Source: CAD feature listing. Evaluate the final solid. Frame: model axes, mm. A direction names the side the tool comes from. Give positions to 0.01 mm unless a question says otherwise; leave off trailing zeros. Order: outer loops, then holes, each group sorted by start corner. A loop starts at its lowest first (then second) coordinate and runs counter-clockwise, first axis right, second up.
```python
from build123d import *

# Parameters (mm, degrees)
BOSS_EXTRUDE1_DEPTH = 9.75
BOSS_EXTRUDE2_START = -1
BOSS_EXTRUDE2_DEPTH = 5
BOSS_EXTRUDE3_START = 1
SKETCH3_R           = 1.6
BOSS_EXTRUDE3_DEPTH = 1
BOSS_EXTRUDE4_DEPTH = 0.5


with BuildPart() as part:
    # Sketch1 → Boss-Extrude1 (new body)
    with BuildSketch(Plane(origin=(0, 0, 0), x_dir=(0, 0, -1), z_dir=(1, 0, 0))):
        Polygon((-4.875, -6.875), (-4.875, 5.125), (4.875, 5.125), (4.875, -6.875), (6.625, -6.875), (6.625, 6.875), (-6.625, 6.875), (-6.625, -6.875), align=None)
    extrude(amount=BOSS_EXTRUDE1_DEPTH)

    # Sketch2 → Boss-Extrude2 (add)
    with BuildSketch(Plane.XZ.offset(6.875).offset(BOSS_EXTRUDE2_START)):
        with BuildLine():
            Line((0, 9.925), (0, 4.875))
            Line((0, 4.875), (7.75, 4.875))
            Line((7.75, 4.875), (7.75, 9.925))
            ThreePointArc((7.75, 9.925), (3.875, 13.8), (0, 9.925))
        make_face()
        Polygon((0.584103466, 9.925), (2.229551733, 12.775), (5.520448267, 12.775), (7.165896534, 9.925), (5.520448267, 7.075), (2.229551733, 7.075), align=None, mode=Mode.SUBTRACT)
    boss_extrude2 = extrude(amount=-BOSS_EXTRUDE2_DEPTH)

    # Sketch3 → Boss-Extrude3 (add)
    with BuildSketch(Plane.XZ.offset(5.875).offset(BOSS_EXTRUDE3_START)):
        with BuildLine():
            Line((7.75, 6.625), (7.75, 9.925))
            ThreePointArc((7.75, 9.925), (3.875, 13.8), (0, 9.925))
            Line((0, 9.925), (0, 6.625))
            Line((0, 6.625), (7.75, 6.625))
        make_face()
        with Locations(Location((3.875, 9.925, 0), (0, 0, 90))):
            Circle(SKETCH3_R, mode=Mode.SUBTRACT)
    boss_extrude3 = extrude(amount=-BOSS_EXTRUDE3_DEPTH)

    # Mirror1: Boss-Extrude2, Boss-Extrude3 across plane
    add(boss_extrude2.mirror(Plane.XY))
    add(boss_extrude3.mirror(Plane.XY))

    # Sketch4 → Boss-Extrude4 (add)
    with BuildSketch(Plane.ZY):
        Polygon((-6.625, 6.875), (-6.625, -6.875), (-4.375, -6.875), (-4.375, 4.625), (4.375, 4.625), (4.375, -6.875), (6.625, -6.875), (6.625, 6.875), align=None)
    extrude(amount=-BOSS_EXTRUDE4_DEPTH)


solid = part.part
```
1) Section query B-B, the plane x = 5. Return the cut outline in (y, z) (3 decimals), and give its area (3 significant figures).
Report:
outline: (-6.875, -13.633) - (-0.875, -13.633) - (-0.875, -12.775) - (-5.875, -12.775) - (-5.875, -11.063) - (-6.875, -11.063) - close; (-6.875, -8.787) - (-5.875, -8.787) - (-5.875, -7.075) - (-0.875, -7.075) - (-0.875, -6.625) - (6.875, -6.625) - (6.875, 6.625) - (-0.875, 6.625) - (-0.875, 7.075) - (-5.875, 7.075) - (-5.875, 8.787) - (-6.875, 8.787) - (-6.875, 4.875) - (5.125, 4.875) - (5.125, -4.875) - (-6.875, -4.875) - close; (-6.875, 11.063) - (-5.875, 11.063) - (-5.875, 12.775) - (-0.875, 12.775) - (-0.875, 13.633) - (-6.875, 13.633) - close
area: 87.7 mm2
2) Material intervals for L1, parallel to Z at x = 0.75, y = 3 (3 decimals); L2, parallel to Y at x = 6, z = 4 (3 decimals); L3, parallel to Y at x = 2, z = 9 (3 decimals), sorted ascending.
Report:
L1: z = -6.625 to -4.875, 4.875 to 6.625
L2: y = 5.125 to 6.875
L3: y = -6.875 to -5.875
3) Section query A-A, the plane y = -2.75. Return the cut outline in (x, z) (3 decimals).
Report:
outline: (0, -9.925) arc R3.875 ccw to (7.75, -9.925) - (7.75, -6.625) - (9.75, -6.625) - (9.75, -4.875) - (0.5, -4.875) - (0.5, -4.375) - (0, -4.375) - close; (0, 4.375) - (0.5, 4.375) - (0.5, 4.875) - (9.75, 4.875) - (9.75, 6.625) - (7.75, 6.625) - (7.75, 9.925) arc R3.875 ccw to (0, 9.925) - close; hole (0.584, -9.925) - (2.23, -12.775) - (5.52, -12.775) - (7.166, -9.925) - (5.52, -7.075) - (2.23, -7.075) - close; hole (0.584, 9.925) - (2.23, 7.075) - (5.52, 7.075) - (7.166, 9.925) - (5.52, 12.775) - (2.23, 12.775) - close
4) Draft query along Z for faces 1 (the flat face through (7.75, -4, -8)), 2 (the cylindrical face through (2.29, -6.38, -9.72)). Return one class per face: +Z half, -Z half, draft (parallel to the pull), parting line (faces both ways), or undercut.
Report:
face 1: draft
face 2: undercut
5) Reachability of faces 3 (the flat face through (1, -0.875, -11)), 4 (the flat face through (4, -3, 12.775)), 5 (the flat face through (0.5, 4.9, 0)) from +Z, -Z, +X, -X, +Y, -Y: full face, straight path, thin tool, end or side. Return the list, or none.
Report:
face 3: -Z, +X, -X, +Y
face 4: +Y
face 5: +X, -Y
6) Pin query (flat end, axial travel): pin 1 (4 mm diameter, centred on x = 8.5, y = -1.5, fed in from -Z); pin 2 (3 mm diameter, centred on x = 5, z = 10.5, fed in from +Y) (3 decimals); pin 3 (0.6 mm diameter, centred on x = 0, y = 0, fed in from -Z) (3 decimals); pin 4 (3 mm diameter, centred on y = -0.5, z = 1, fed in from +X). Return the tip coordinate at first contact, or that it passes through.
Report:
pin 1: stops at z = -12.78
pin 2: stops at y = -5.875
pin 3: stops at z = -6.625
pin 4: passes through
7) Section query C-C, the plane y = 2.75. Return the cut outline in (x, z) (3 decimals).
Report:
outline: (0, -6.625) - (9.75, -6.625) - (9.75, -4.875) - (0.5, -4.875) - (0.5, -4.375) - (0, -4.375) - close; (0, 4.375) - (0.5, 4.375) - (0.5, 4.875) - (9.75, 4.875) - (9.75, 6.625) - (0, 6.625) - close
8) Section query D-D, the plane z = 10.5. Return the cut outline in (x, y) (3 decimals).
Report:
outline: (0.043, -6.875) - (2.382, -6.875) - (2.382, -5.875) - (0.916, -5.875) - (0.916, -0.875) - (0.043, -0.875) - close; (5.368, -6.875) - (7.707, -6.875) - (7.707, -0.875) - (6.834, -0.875) - (6.834, -5.875) - (5.368, -5.875) - close
